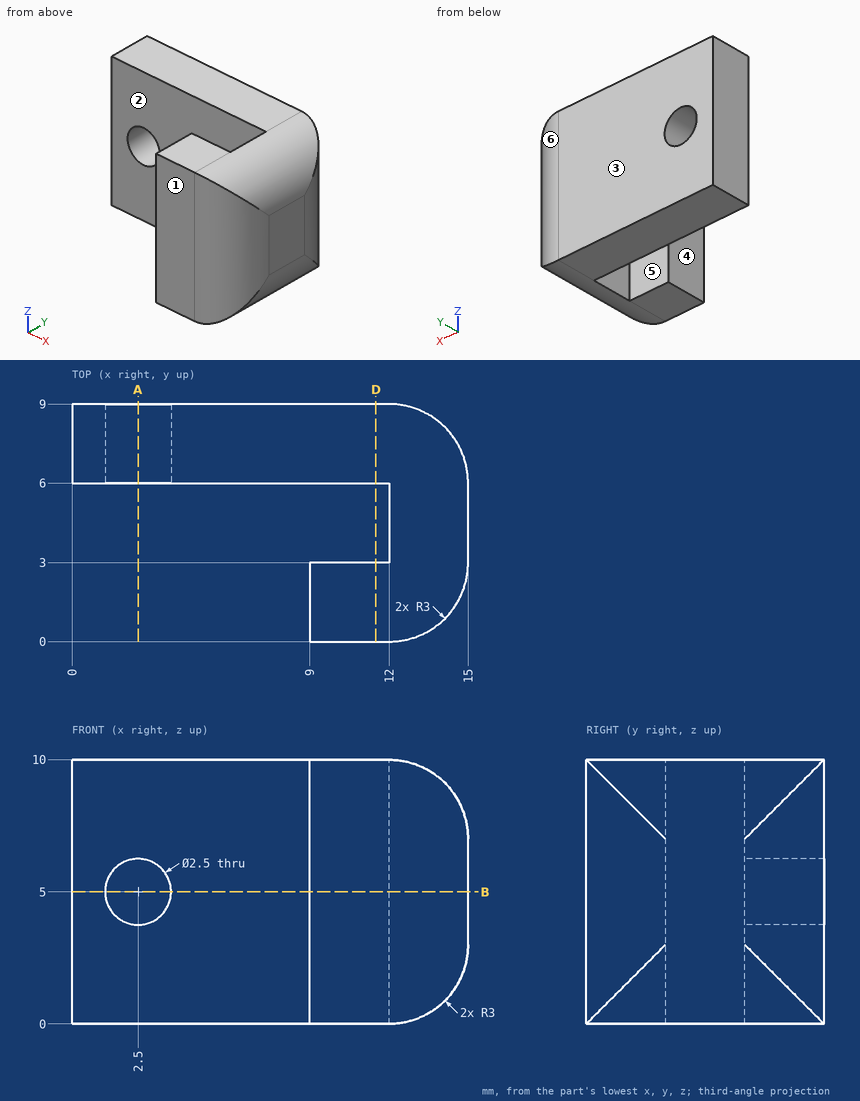
Input: dimensioned drawing with shaded views. Units: mm. Origin: part minimum x, y, z. A direction names the side the tool comes from. Give positions to 0.01 mm unless a question says otherwise; leave off trailing zeros. Write each loop counter-clockwise with the first axis right and the second up, starting at its lowest first coordinate (ties: lowest second). Pieces come first, ordered by that corner, then holes. Notation, with made-up numbers: (25, 60) - (80, 60) arc R16 cw to (80, 86) - close; hole circle Ø4 at (15, -39). An arc over 180 degrees is marked (long way). One line per item, written item: value. Start each with the question number.
Q1. Section query D-D, the plane x = 11.5. Return the cut outline in (y, z).
Q2. Material intervals for probe 1 along Z at (x, y) = (2.5, 7); probe 2 along Y at (x, z) = (11.25, 4); probe 3 along Y at (x, z) = (4, 4.5), sorted ascending. Write a range as from..to.
Q3. First-contact query: pin 1 Ø0.9 at (y, z) = (4, 5.5) entering from -X; pin 2 Ø3 at (x, z) = (3.5, 2.5) entering from -Y; pin 3 Ø0.9 at (y, z) = (1.5, 3.5) entering from -X. Flat tips, straight axial feed; report the tip coordinate or a pass-through.
Q4. Set-up query: the marked faces 4, 5 and 6. Return all of +Z, -Z, +X, -X, +Y, -Y with unobstructed straight access to the full face (end or side cutting, diameter ignored); none if empty.
Q5. Section query B-B, the plane z = 5. Return the cut outline in (x, y), then the cut area to 3 significant figures.
Q6. Draft query along Y for the marked faces 1, 2 and 3. Return one class per face: +Y half, -Y half, draft (parallel to the pull), parting line (faces both ways), or undercut.
Q7. Section query A-A, the plane x = 2.5. Return the cut outline in (y, z), then the cut area to 3 significant figures.
Answer:
1. outline: (0, 0) - (3, 0) - (3, 10) - (0, 10) - close; (6, 0) - (9, 0) - (9, 10) - (6, 10) - close
2. probe 1: z = 0..3.75, 6.25..10
2. probe 2: y = 0..3, 6..9
2. probe 3: y = 6..9
3. pin 1: stops at x = 12
3. pin 2: stops at y = 6
3. pin 3: stops at x = 9
4. face 4: +Z, -Z, -X, -Y
4. face 5: +Z, -Z, -X
4. face 6: +Z, -Z, +X, +Y
5. outline: (0, 6) - (1.25, 6) - (1.25, 9) - (0, 9) - close; (3.75, 6) - (12, 6) - (12, 3) - (9, 3) - (9, 0) - (12, 0) arc R3 ccw to (15, 3) - (15, 6) arc R3 ccw to (12, 9) - (3.75, 9) - close
5. area: 60.6 mm2
6. face 1: -Y half
6. face 2: undercut
6. face 3: +Y half
7. outline: (6, 0) - (9, 0) - (9, 3.75) - (6, 3.75) - close; (6, 6.25) - (9, 6.25) - (9, 10) - (6, 10) - close
7. area: 22.5 mm2
